Drawing for the job (mm, zero at the part's lowest x, y, z). A direction names the side the tool comes from. Coordinates: 2 decimals unless noted, no trailing zeros. Write each loop counter-clockwise with the first axis right and the second up, starting at its lowest first coordinate (ties: lowest second). Pieces come first, ordered by that corner, then holes. Notation, with made-up numbers: (-9.75, 57) -> (36.25, 57) arc R8 cw to (36.25, 70) -> close; hole circle Ø2 at (3, 61). An arc over 180 degrees is marked (long way). Write item = value, one per line. Start each with the question number.
Q1. Band-saw the part on C-C, the plane x = 42. List the corners of the cut face in (y, z).
Q2. Tool access for the marked faces 1 and 2: list every direction of +Z, -Z, +X, -X, +Y, -Y with a clear straight run to the whole face (end or side of a thin tool).
Q3. Band-saw the part on B-B, the plane z = 14. List the corners of the cut face in (x, y), plus the area to 3 significant figures.
Q4. Pull direction X, two halves, no side cores. Call the marked faces 3, 4 and 5: released by +X, released by -X, zero draft, split by the parting line, or undercut.
Q5. Band-saw the part on A-A, the plane x = 54.5. List the corners of the cut face in (y, z).
Q6. Probe line 1 (X direction, y = 9.4, z = 2.9); line 2 (Z direction, x = 2.5, y = 8.85); line 3 (Z direction, x = 20.5, y = 7.5). List the from-to ranges inside material, lowest first.
Q7. Pin check, flat tips, straight feed: P1, Ø2, axis at x = 3.5, y = 11.5, coming from the +Z side; P2, Ø1.2, axis at y = 11, z = 14.5, coming from the +X side; P3, Ø2.5, axis at x = 54.5, z = 2.9, coming from the -Y side; P4, Ø9, axis at x = 32, z = 9, coming from the -Y side. Stop position of each tip, or through.
Q8. Band-saw the part on D-D, the plane x = 2.5. List the corners of the cut face in (y, z), plus the area to 3 significant figures.
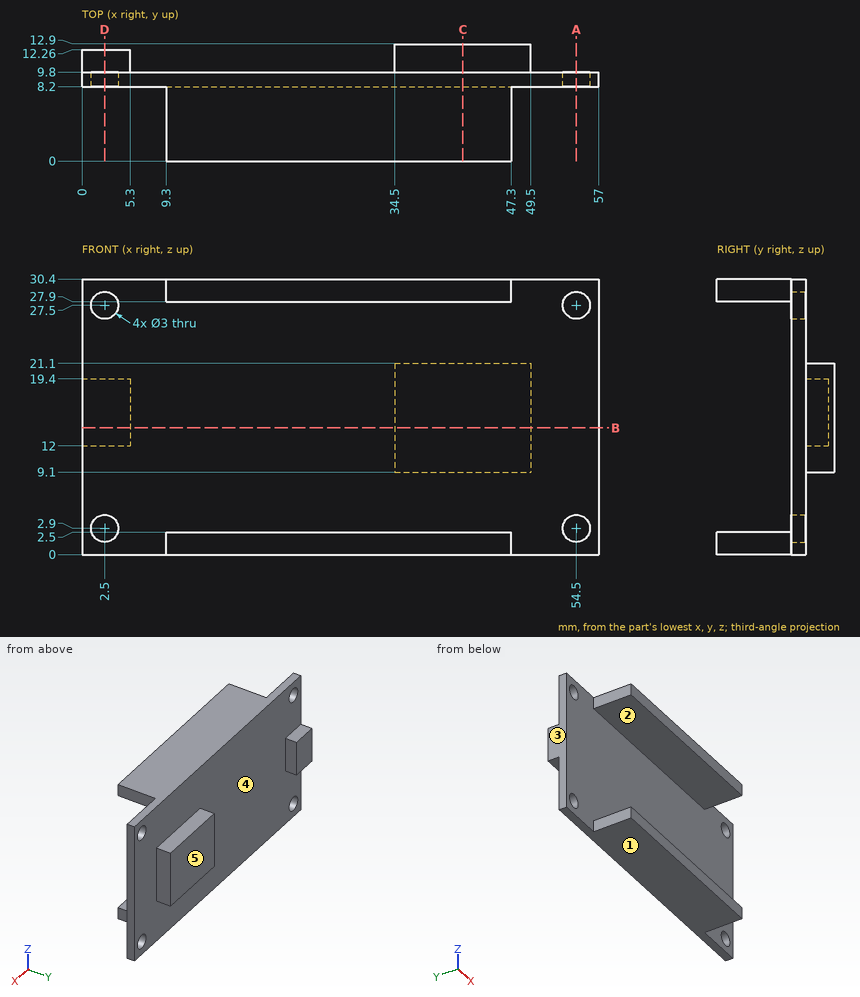
Ans:
q1.outline = (0, 0) -> (9.8, 0) -> (9.8, 9.1) -> (12.9, 9.1) -> (12.9, 21.1) -> (9.8, 21.1) -> (9.8, 30.4) -> (0, 30.4) -> (0, 27.9) -> (8.2, 27.9) -> (8.2, 2.5) -> (0, 2.5) -> close
q2.face_1 = -Z, +X, -X, +Y, -Y
q2.face_2 = +X, -X, -Y
q3.outline = (0, 8.2) -> (57, 8.2) -> (57, 9.8) -> (49.5, 9.8) -> (49.5, 12.9) -> (34.5, 12.9) -> (34.5, 9.8) -> (5.3, 9.8) -> (5.3, 12.26) -> (0, 12.26) -> close
q3.area = 151 mm2
q4.face_3 = released by -X
q4.face_4 = undercut
q4.face_5 = zero draft
q5.outline = (8.2, 0) -> (9.8, 0) -> (9.8, 1.4) -> (8.2, 1.4) -> close; (8.2, 4.4) -> (9.8, 4.4) -> (9.8, 26) -> (8.2, 26) -> close; (8.2, 29) -> (9.8, 29) -> (9.8, 30.4) -> (8.2, 30.4) -> close
q6.line_1 = 0 to 1, 4 to 53, 56 to 57
q6.line_2 = 0 to 1.4, 4.4 to 26, 29 to 30.4
q6.line_3 = 0 to 2.5, 27.9 to 30.4
q7.P1 = 19.4
q7.P2 = 49.5
q7.P3 = through
q7.P4 = 8.2
q8.outline = (8.2, 0) -> (9.8, 0) -> (9.8, 1.4) -> (8.2, 1.4) -> close; (8.2, 4.4) -> (9.8, 4.4) -> (9.8, 12) -> (12.26, 12) -> (12.26, 19.4) -> (9.8, 19.4) -> (9.8, 26) -> (8.2, 26) -> close; (8.2, 29) -> (9.8, 29) -> (9.8, 30.4) -> (8.2, 30.4) -> close
q8.area = 57.2 mm2
